For this review, take the finished solid that the model builds, in its own axes (mm). A direction names the side the tool comes from. Give positions to 0.01 mm unless a question says otherwise; leave off trailing zeros. Loops run counter-clockwise (first coordinate to the right, second up) from the corner with the lowest first, then second, coordinate; pieces in that order, holes last. Notation, with made-up numbers: (89.5, 75.5) - (94.5, 75.5) arc R29 ccw to (94.5, 113.5) - close; hole circle Ø8 at (54.25, 61). An arc over 180 degrees is marked (long way). Use CSV: the item, a comma, the result in double quotes. Start each with the question number.
1. Mouldability with a two-part tool opening along Y and no side actions: class faces 1 (the cylindrical face through (-20.63, 31.94, 0.16)), 2 (the cylindrical face through (-0.51, 21.51, 0.99)), 3 (the flat face through (1, 0, 4)), 4 (the cylindrical face through (-35.198, 11.063, 16.097)) as pulls with the +Y half, pulls with the -Y half, needs draft (parallel to the pull), parting line crosses it, or undercut.
2. Take a section at B-B on z = 16. Give the boundary of the cut face in (x, y), plus the area to 3 significant figures.
3. For pin 1 (5.5 mm diameter, centred on x = -16.5, z = 7, fed in from +Y); pin 2 (5 mm diameter, centred on y = 18.5, z = 15, fed in from -X); pin 3 (10 mm diameter, centred on x = -2, z = 8, fed in from -Y); pin 4 (2.5 mm diameter, centred on x = -15.5, y = 17.5, fed in from -Z), all flat-tipped, find the tip position at first contact; note any pin that passes through.
4. For faces 5 (the cylindrical face through (31.801, 11.459, 21.487)), 6 (the flat face through (-23, 22, 11)), 7 (the cylindrical face through (-22.459, 23.534, 21.487)), 8 (the cylindrical face through (30.913, 11.459, 0.513)), list the 3-axis set-ups (+Z, -Z, +X, -X, +Y, -Y) from which the entire face can be reached by the end or side of a thin tool; tool diameter is ignored.
5. Take a section at D-D on x = -33. Give the boundary of the cut face in (y, z).
6. Take a section at A-A on x = 15.5. Give the boundary of the cut face in (y, z), plus the area to 3 significant figures.
7. Take a section at C-C on y = 26. Give the boundary of the cut face in (x, z).
8. Wall thickness on line 1 (X direction, y = 14, z = 3.25); line 2 (Y direction, x = -15.5, z = 0.6); line 3 (X direction, y = 48.5, z = 0.6): over which ranges is each line inside the solid? List them lowest first.
```python
from build123d import *
from build123d import SkipClean  # not in build123d's __all__

# Parameters (mm, degrees)
F1_DEPTH  = 2
F3_DEPTH  = 2
F5_DEPTH  = 18
F6_W      = 39
F6_H      = 1.9
F7_DEPTH  = 5
F9_D      = 3.3
F9_DEPTH  = 8
F9_TIP    = 0.9914200214
F11_D     = 4.4
F11_DEPTH = 8
F11_TIP   = 1.3218933619
F12_R     = 1.8


with BuildPart() as f1:
    # F0 (on Top) → F1 (new body)
    with BuildSketch(Plane.XY):
        with BuildLine():
            Line((0, 21.5), (0, 0))
            Line((0, 0), (39, 0))
            Line((39, 0), (39, 12))
            Line((39, 12), (23, 12))
            Line((23, 12), (23, 33))
            Line((23, 33), (21, 33))
            Line((21, 33), (21, 51))
            Line((21, 51), (18, 54))
            Line((18, 54), (0, 54))
            Line((0, 54), (0, 44.5))
            ThreePointArc((0, 44.5), (11.5, 33), (0, 21.5))
        make_face()
    extrude(amount=F1_DEPTH)

    # F2 (on face) → F3 (join)
    with BuildSketch(Plane.XY.offset(2)):
        Polygon((0, 12), (0, 0), (39, 0), (39, 12), (23, 12), (23, 33), (21.1, 33), (21.1, 12), align=None)
    extrude(amount=F3_DEPTH)

    # F4 (on face) → F5 (join)
    with BuildSketch(Plane.XY.offset(4)):
        Polygon((23, 33), (21.1, 33), (21.1, 12), (0, 12), (0, 10.1), (39, 10.1), (39, 12), (23, 12), align=None)
    extrude(amount=F5_DEPTH)

    # F6 (on face) → F7 (join)
    with BuildSketch(Plane.XY.offset(4)):
        with Locations((19.5, 0.95)):
            Rectangle(F6_W, F6_H)
    extrude(amount=F7_DEPTH)

    # F9
    with Locations(Plane(origin=(0, 0, 0), x_dir=(1, 0, 0), z_dir=(0, 0, -1))):
        with Locations((15.5, -17.5), (15.5, -48.5)):
            Hole(F9_D / 2, depth=F9_DEPTH)
            with Locations((0, 0, -(F9_DEPTH + F9_TIP / 2))):  # 118° drill point
                Cone(0, F9_D / 2, F9_TIP, mode=Mode.SUBTRACT)

    # F11
    with Locations(Plane.XZ.offset(-10.1)):
        with Locations((33, 16)):
            Hole(F11_D / 2, depth=F11_DEPTH)
            with Locations((0, 0, -(F11_DEPTH + F11_TIP / 2))):  # 118° drill point
                Cone(0, F11_D / 2, F11_TIP, mode=Mode.SUBTRACT)

    # F12
    f12_edges = [f1.edges().sort_by_distance(p)[0] for p in [
        (31, 12, 22),
        (39, 12, 11),
        (23, 33, 11),
        (23, 22.5, 22),
        (23, 22.5, 0),
        (9, 54, 0),
        (31, 12, 0),
        (23, 12, 11),
        (39, 6, 0),
        (19.5, 0, 9),
        (19.5, 0, 0),
        (39, 0, 4.5),
        (21, 42, 0),
        (22, 33, 0),
        (19.5, 52.5, 0),
    ]]
    fillet(f12_edges, radius=F12_R)

    # F13: F1 across plane


with BuildPart() as f1_1:
    add(f1.part, clean=False)
    with SkipClean():  # cleaning this boolean's faces spoils the solid; the shape is the same uncleaned
        add(f1.part.mirror(Plane.YZ), clean=False)


solid = f1_1.part
```
Check result:
1,face 1,"pulls with the +Y half"
1,face 2,"undercut"
1,face 3,"pulls with the -Y half"
1,face 4,"needs draft"
2,outline,"(-39, 10.1) - (-35.2, 10.1) - (-35.2, 12) - (-37.2, 12) arc R1.8 ccw to (-39, 10.2) - close; (-30.8, 10.1) - (30.8, 10.1) - (30.8, 12) - (24.8, 12) arc R1.8 cw to (23, 13.8) - (23, 31.2) arc R1.8 ccw to (21.2, 33) - (21.1, 33) - (21.1, 12) - (-21.1, 12) - (-21.1, 33) - (-21.2, 33) arc R1.8 ccw to (-23, 31.2) - (-23, 13.8) arc R1.8 cw to (-24.8, 12) - (-30.8, 12) - close; (35.2, 10.1) - (39, 10.1) - (39, 10.2) arc R1.8 ccw to (37.2, 12) - (35.2, 12) - close"
2,area,"210 mm²"
3,pin 1,"stops at y = 12"
3,pin 2,"stops at x = -23"
3,pin 3,"stops at y = 0"
3,pin 4,"passes through"
4,face 5,"+Z, +X, +Y"
4,face 6,"+Z, -Z, -X, +Y"
4,face 7,"+Z, -X, +Y"
4,face 8,"-Z, +X, +Y"
5,outline,"(0, 1.8) arc R1.8 ccw to (1.8, 0) - (10.2, 0) arc R1.8 ccw to (12, 1.8) - (12, 13.8) - (10.1, 13.8) - (10.1, 4) - (1.9, 4) - (1.9, 9) - (1.8, 9) arc R1.8 ccw to (0, 7.2) - close; (10.1, 18.2) - (12, 18.2) - (12, 20.2) arc R1.8 ccw to (10.2, 22) - (10.1, 22) - close"
6,outline,"(0, 1.8) arc R1.8 ccw to (1.8, 0) - (15.85, 0) - (15.85, 2) - (12, 2) - (12, 22) - (10.1, 22) - (10.1, 4) - (1.9, 4) - (1.9, 9) - (1.8, 9) arc R1.8 ccw to (0, 7.2) - close; (19.15, 0) - (46.85, 0) - (46.85, 2) - (19.15, 2) - close; (50.15, 0) - (52.2, 0) arc R1.8 ccw to (54, 1.8) - (54, 2) - (50.15, 2) - close"
6,area,"160 mm²"
7,outline,"(-23, 1.8) arc R1.8 ccw to (-21.2, 0) - (-9.12, 0) - (-9.12, 2) - (-21.1, 2) - (-21.1, 22) - (-21.2, 22) arc R1.8 ccw to (-23, 20.2) - close; (9.12, 0) - (21.2, 0) arc R1.8 ccw to (23, 1.8) - (23, 20.2) arc R1.8 ccw to (21.2, 22) - (21.1, 22) - (21.1, 2) - (9.12, 2) - close"
8,line 1,"x = -23 to -21.1, 21.1 to 23"
8,line 2,"y = 0.46 to 15.85, 19.15 to 46.85, 50.15 to 53.54"
8,line 3,"x = -20.54 to -17.15, -13.85 to 13.85, 17.15 to 20.54"
